from build123d import *

# Parameters (mm, degrees)
SKETCH017_W               = 60
SKETCH017_H               = 44
EXTRUDE021_DEPTH          = 2
CHAMFER001_SIZE           = 1.5
EXTRUDE024_DEPTH          = 8
SKETCH016_R               = 4
EXTRUDE020_DEPTH          = 49
FUSION008_PLACEMENT_ANGLE = 180


with BuildPart() as chamfer001:
    # Sketch017 (on Extrude) → Extrude021 (new body, symmetric)
    with BuildSketch(Plane.XZ):
        with Locations((-30, 26)):
            Rectangle(SKETCH017_W, SKETCH017_H)
    extrude(amount=EXTRUDE021_DEPTH, both=True)

    # Chamfer001
    chamfer001_edges = [chamfer001.edges().sort_by_distance(p)[0] for p in [
        (-60, 2, 26),
        (-60, -2, 26),
    ]]
    chamfer(chamfer001_edges, length=CHAMFER001_SIZE)


with BuildPart() as extrude024:
    # Sketch019 → Extrude024 (new body)
    with BuildSketch(Plane.XY):
        Polygon((-1.5, 2.598076), (1.5, 2.598076), (3, 0), (1.5, -2.598076), (-1.5, -2.598076), (-3, 0), align=None)
    extrude(amount=-EXTRUDE024_DEPTH)


with BuildPart() as reject_flap:
    # Sketch016 → Extrude020 (new body)
    with BuildSketch(Plane.XY):
        Circle(SKETCH016_R)
    extrude(amount=EXTRUDE020_DEPTH)

    # Fusion008: union Chamfer001, Extrude024
    add(chamfer001.part)
    add(extrude024.part)


with BuildPart() as reject_flap_1:
    # Fusion008 placement: moved
    add(reject_flap.part.rotate(Axis((0, 0, 0), (0, 1, 0)), FUSION008_PLACEMENT_ANGLE))


solid = reject_flap_1.part
Could you check a few things on this model? Use its own coordinates, in mm. A direction names the side the tool comes from. Coordinates: 2 decimals unless noted, no trailing zeros. Write each loop counter-clockwise with the first axis right and the second up, starting at its lowest first coordinate (ties: lowest second). Pieces come first, ordered by that corner, then holes. Notation, with made-up numbers: (43, 84) - (84, 84) arc R16 ccw to (84, 89) - close; hole circle Ø9 at (-22.5, 9.25). An arc over 180 degrees is marked (long way). Write item = value, one per line.
1) For faces 1 (the flat face through (32, 0, -48)), 2 (the flat face through (2.24, -1.32, 3.94)), 3 (the flat face through (31, -2, -26)), which set-ups out of +Z, -Z, +X, -X, +Y, -Y let a thin tool reach every point of the face, with its end or its side?
Result set:
face_1 = -Z, +X, +Y, -Y
face_2 = +Z, +X, -Y
face_3 = +Z, -Z, +X, -Y
2) Suppose I cut it at B-B on z = -35. Please give me the cut outline in (x, y).
Result set:
outline = (3.46, -2) - (58.5, -2) - (60, -0.5) - (60, 0.5) - (58.5, 2) - (3.46, 2) arc R4 ccw (long way) to start
3) Suppose I cut it at C-C on x = 40.5. Please give me the cut outline in (y, z).
Result set:
outline = (-2, -48) - (2, -48) - (2, -4) - (-2, -4) - close
4) Will these pins go through, and if not, where does the flat tip stop? pin 1 Ø22 at (x, z) = (40, -20.5) entering from -Y; pin 2 Ø8 at (x, z) = (28.5, -7.5) entering from +Y; pin 3 Ø1.5 at (x, z) = (0, 2) entering from -Y.
Result set:
pin_1 = -2
pin_2 = 2
pin_3 = -2.6
5) Please list where these lines run through material, in increasing order: line 1 (Z direction, x = 28, y = -1.25); line 2 (Y direction, x = 44, z = -34); line 3 (X direction, y = 0.25, z = -39). Write a range as [from, to].
Result set:
line_1 = [-48, -4]
line_2 = [-2, 2]
line_3 = [-3.99, 60]
6) Suppose I cut it at A-A on x = 0. Please give me the cut outline in (y, z).
Result set:
outline = (-4, -49) - (4, -49) - (4, 0) - (2.6, 0) - (2.6, 8) - (-2.6, 8) - (-2.6, 0) - (-4, 0) - close
